The model under review builds one solid part; all positions refer to its coordinate system, in mm. Face numbers are marked on the shaded views. A direction names the side the tool comes from. Give positions to 0.01 mm unless a question says otherwise; leave off trailing zeros. Order: outer loops, then holes, each group sorted by start corner. A loop starts at its lowest first (then second) coordinate and runs counter-clockwise, first axis right, second up. Notation, with made-up numbers: (45, -21) - (79, -21) arc R16 ccw to (79, -15) - close; hole circle Ø10 at (-4, -34.5). An arc over 180 degrees is marked (long way). Put each result on its own line as item: value.
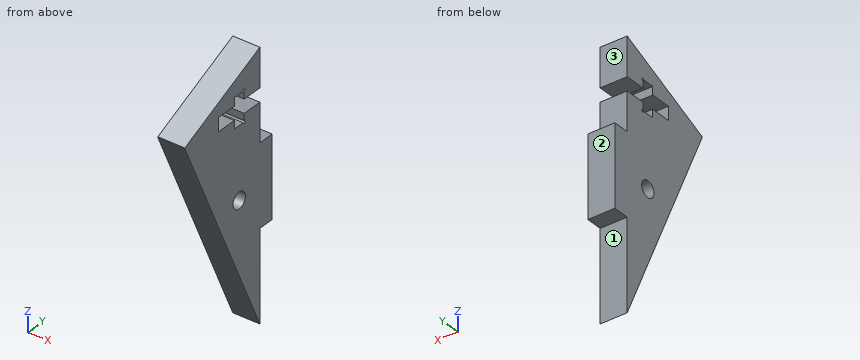
```python
from build123d import *

# Parameters (mm, degrees)
SCHIZZO1_W                   = 48.55
SCHIZZO1_H                   = 18.21
ESTRUSIONE_ESTRUSIONE1_DEPTH = 5
TAGLIO_ESTRUSIONE1_DEPTH     = 6
SCHIZZO3_R                   = 1.5
TAGLIO_ESTRUSIONE2_DEPTH     = 6
SCHIZZO4_W                   = 5
SCHIZZO4_H                   = 15
ESTRUSIONE_ESTRUSIONE2_DEPTH = 3
TAGLIO_ESTRUSIONE3_DEPTH     = 6
SCHIZZO7_R                   = 0.25
TAGLIO_ESTRUSIONE4_DEPTH     = 6


with BuildPart() as part:
    # Schizzo1 → Estrusione-Estrusione1 (new body)
    with BuildSketch(Plane(origin=(0, 0, 0), x_dir=(0, 0, -1), z_dir=(1, 0, 0))):
        Rectangle(SCHIZZO1_W, SCHIZZO1_H)
    extrude(amount=ESTRUSIONE_ESTRUSIONE1_DEPTH)

    # Schizzo2 → Taglio-Estrusione1 (cut, through all)
    with BuildSketch(Plane(origin=(0, 0, 0), x_dir=(0, 0, -1), z_dir=(1, 0, 0))):
        Polygon((24.275, 9.105), (-15.905998409, -9.105), (24.275, -9.105), align=None)
        Polygon((-24.275, 9.105), (-24.275, -9.105), (-16.019269678, -9.111556119), align=None)
    extrude(amount=TAGLIO_ESTRUSIONE1_DEPTH, mode=Mode.SUBTRACT)

    # Schizzo3 → Taglio-Estrusione2 (cut, through all)
    with BuildSketch(Plane(origin=(0, 0, 0), x_dir=(0, 0, -1), z_dir=(1, 0, 0))):
        with Locations((0, 4.105)):
            Circle(SCHIZZO3_R)
    extrude(amount=TAGLIO_ESTRUSIONE2_DEPTH, mode=Mode.SUBTRACT)

    # Schizzo4 → Estrusione-Estrusione2 (add)
    with BuildSketch(Plane(origin=(0, 9.105, 0), x_dir=(1, 0, 0), z_dir=(0, 1, 0))):
        with Locations((2.5, 0)):
            Rectangle(SCHIZZO4_W, SCHIZZO4_H)
    extrude(amount=ESTRUSIONE_ESTRUSIONE2_DEPTH)

    # Schizzo6 → Taglio-Estrusione3 (cut, through all)
    with BuildSketch(Plane(origin=(0, 0, 0), x_dir=(0, 0, -1), z_dir=(1, 0, 0))):
        Polygon((-17.1375, -0.895), (-17.1375, 2.905), (-18.6375, 2.905), (-18.6375, 5.305), (-17.1375, 5.305), (-17.1375, 9.105), (-14.6375, 9.105), (-14.6375, 5.305), (-13.1375, 5.305), (-13.1375, 2.905), (-14.6375, 2.905), (-14.6375, -0.895), align=None)
    extrude(amount=TAGLIO_ESTRUSIONE3_DEPTH, mode=Mode.SUBTRACT)

    # Schizzo7 → Taglio-Estrusione4 (cut, through all)
    with BuildSketch(Plane(origin=(5, 0, 0), x_dir=(0, 0, -1), z_dir=(1, 0, 0))):
        with Locations((-18.6375, 5.305)):
            Circle(SCHIZZO7_R)
        with Locations((-13.1375, 5.305)):
            Circle(SCHIZZO7_R)
    extrude(amount=-TAGLIO_ESTRUSIONE4_DEPTH, mode=Mode.SUBTRACT)


solid = part.part
```
(1) Wall thickness on L1, parallel to Z at x = 4.3, y = 4; L2, parallel to Y at x = 2, z = 0 (3 decimals); L3, parallel to Z at x = 2.4, y = 4.5: over which ranges is each line inside the solid? List them lowest first.
The answers:
L1: -13.01 to -1.5, 1.5 to 13.14, 18.64 to 21.96
L2: -1.896 to 2.605, 5.605 to 12.105
L3: -14.11 to -1.45, 1.45 to 13.14, 18.64 to 22.19
(2) Clearance check with flat-ended pins moving along their axes: pin 1 Ø3 at (x, y) = (2, 0) entering from -Z; pin 2 Ø0.6 at (x, y) = (3.5, 4) entering from -Z; pin 3 Ø1 at (x, z) = (1.5, 17.5) entering from -Y. State where each tip first meets the part, or that it passes through.
The answers:
pin 1: z = -7.49
pin 2: z = -13.67
pin 3: y = -6.95
(3) For the marked faces 1, 2 and 3, list the 3-axis set-ups (+Z, -Z, +X, -X, +Y, -Y) from which the entire face can be reached by the end or side of a thin tool; tool diameter is ignored.
The answers:
face 1: -Z, +X, -X, +Y
face 2: +Z, -Z, +X, -X, +Y
face 3: +Z, +X, -X, +Y
(4) Take a section at A-A, the plane z = 0. Write out the cut boundary in (x, y) (3 decimals).
The answers:
outline: (0, -1.896) - (5, -1.896) - (5, 2.605) - (0, 2.605) - close; (0, 5.605) - (5, 5.605) - (5, 12.105) - (0, 12.105) - close
(5) Take a section at B-B, the plane y = 1.25. Write out the cut boundary in (x, z).
The answers:
outline: (0, -6.94) - (5, -6.94) - (5, 14.64) - (0, 14.64) - close; (0, 17.14) - (5, 17.14) - (5, 20.72) - (0, 20.72) - close
(6) Take a section at D-D, the plane z = -7. Write out the cut boundary in (x, y) (3 decimals), then the cut area to 3 significant figures.
The answers:
outline: (0, 1.276) - (5, 1.276) - (5, 12.105) - (0, 12.105) - close
area: 54.1 mm^2
